The listing builds one solid part. Answer for the finished solid, in the listing's coordinates (mm). Face numbers are marked on the shaded views. A direction names the side the tool comes from. Round coordinates to 2 decimals unless told otherwise and drop trailing zeros. Order: outer loops, then holes, each group sorted by start corner. A loop starts at its lowest first (then second) coordinate and runs counter-clockwise, first axis right, second up. Notation, with made-up numbers: (-17.75, -38) - (38.25, -38) arc R13 ccw to (38.25, -26) - close; hole circle Ø10 at (-29.75, -34). An arc over 180 degrees is marked (long way). One line per item, written item: value. Start each with the question number.
1. A straight line is drawn through the part: line 1 (Z direction, x = 12, y = 18). Find the intervals that lie inside material, in ascending order.
2. Section A-A, the plane z = 11.5 is taken. Count the separate pieces of the cut face and the enclosed holes in it, then the cut area to 3 significant figures.
3. Section B-B, the plane x = 22 is taken. Give the vertices of the cut face in (y, z).
4. A tool of negligible diameter and unlimited length cuts with its end or side. For the marked faces 1, 2 and 3, from which of +Z, -Z, +X, -X, +Y, -Y can it reach the whole face along a straight path? Write none if from no direction.
5. Flat-ended cylindrical pins translate along their axes: P1, Ø3, axis at y = 20.5, z = 6.5, coming from the -X side; P2, Ø6, axis at y = 4, z = 10, coming from the +X side; P3, Ø0.6, axis at x = 3.5, z = 8, coming from the +Y side. Find the tip coordinate at first contact, or state that the pin passes through.
from build123d import *

# Parameters (mm, degrees)
F0_W     = 0.508
F0_H     = 27.8820712173
F1_DEPTH = 12.7
F0_W_2   = 29.972
F0_H_2   = 29.972
F2_DEPTH = 2.54


with BuildPart() as f1:
    # F0 (on Top) → F1 (new body)
    with BuildSketch(Plane.XY):
        with Locations((0.762, 15.0149643914)):
            Rectangle(F0_W, F0_H)
    extrude(amount=F1_DEPTH)



with BuildPart() as f1b:
    # F0 (on Top) → F1, piece 2 (new body)
    with BuildSketch(Plane.XY):
        with Locations((3.302, 15.0149643914)):
            Rectangle(F0_W, F0_H)
    extrude(amount=F1_DEPTH)


with BuildPart() as f1c:
    # F0 (on Top) → F1, piece 3 (new body)
    with BuildSketch(Plane.XY):
        with Locations((5.842, 15.0149643914)):
            Rectangle(F0_W, F0_H)
    extrude(amount=F1_DEPTH)


with BuildPart() as f1d:
    # F0 (on Top) → F1, piece 4 (new body)
    with BuildSketch(Plane.XY):
        with Locations((8.382, 15.0149643914)):
            Rectangle(F0_W, F0_H)
    extrude(amount=F1_DEPTH)


with BuildPart() as f1e:
    # F0 (on Top) → F1, piece 5 (new body)
    with BuildSketch(Plane.XY):
        with Locations((10.922, 15.0149643914)):
            Rectangle(F0_W, F0_H)
    extrude(amount=F1_DEPTH)


with BuildPart() as f1f:
    # F0 (on Top) → F1, piece 6 (new body)
    with BuildSketch(Plane.XY):
        with Locations((13.462, 15.0149643914)):
            Rectangle(F0_W, F0_H)
    extrude(amount=F1_DEPTH)


with BuildPart() as f1g:
    # F0 (on Top) → F1, piece 7 (new body)
    with BuildSketch(Plane.XY):
        with Locations((16.002, 15.0149643914)):
            Rectangle(F0_W, F0_H)
    extrude(amount=F1_DEPTH)


with BuildPart() as f1h:
    # F0 (on Top) → F1, piece 8 (new body)
    with BuildSketch(Plane.XY):
        with Locations((18.542, 15.0149643914)):
            Rectangle(F0_W, F0_H)
    extrude(amount=F1_DEPTH)


with BuildPart() as f1i:
    # F0 (on Top) → F1, piece 9 (new body)
    with BuildSketch(Plane.XY):
        with Locations((21.082, 15.0149643914)):
            Rectangle(F0_W, F0_H)
    extrude(amount=F1_DEPTH)


with BuildPart() as f1j:
    # F0 (on Top) → F1, piece 10 (new body)
    with BuildSketch(Plane.XY):
        with Locations((23.622, 15.0149643914)):
            Rectangle(F0_W, F0_H)
    extrude(amount=F1_DEPTH)


with BuildPart() as f1k:
    # F0 (on Top) → F1, piece 11 (new body)
    with BuildSketch(Plane.XY):
        with Locations((26.162, 15.0149643914)):
            Rectangle(F0_W, F0_H)
    extrude(amount=F1_DEPTH)


with BuildPart() as f1l:
    # F0 (on Top) → F1, piece 12 (new body)
    with BuildSketch(Plane.XY):
        with Locations((28.702, 15.0149643914)):
            Rectangle(F0_W, F0_H)
    extrude(amount=F1_DEPTH)


with BuildPart() as f1_1:
    add(f1.part)

    add(f1b.part)  # F2 merges F1b

    add(f1c.part)  # F2 merges F1c

    add(f1d.part)  # F2 merges F1d

    add(f1e.part)  # F2 merges F1e

    add(f1f.part)  # F2 merges F1f

    add(f1g.part)  # F2 merges F1g

    add(f1h.part)  # F2 merges F1h

    add(f1i.part)  # F2 merges F1i

    add(f1j.part)  # F2 merges F1j

    add(f1k.part)  # F2 merges F1k

    add(f1l.part)  # F2 merges F1l
    # F0 (on Top) → F2 (join)
    with BuildSketch(Plane.XY):
        with Locations((14.986, 14.986)):
            Rectangle(F0_W_2, F0_H_2)
        with Locations((0.762, 15.0149643914)):
            Rectangle(F0_W, F0_H, mode=Mode.SUBTRACT)
        with Locations((3.302, 15.0149643914)):
            Rectangle(F0_W, F0_H, mode=Mode.SUBTRACT)
        with Locations((5.842, 15.0149643914)):
            Rectangle(F0_W, F0_H, mode=Mode.SUBTRACT)
        with Locations((8.382, 15.0149643914)):
            Rectangle(F0_W, F0_H, mode=Mode.SUBTRACT)
        with Locations((10.922, 15.0149643914)):
            Rectangle(F0_W, F0_H, mode=Mode.SUBTRACT)
        with Locations((13.462, 15.0149643914)):
            Rectangle(F0_W, F0_H, mode=Mode.SUBTRACT)
        with Locations((16.002, 15.0149643914)):
            Rectangle(F0_W, F0_H, mode=Mode.SUBTRACT)
        with Locations((18.542, 15.0149643914)):
            Rectangle(F0_W, F0_H, mode=Mode.SUBTRACT)
        with Locations((21.082, 15.0149643914)):
            Rectangle(F0_W, F0_H, mode=Mode.SUBTRACT)
        with Locations((23.622, 15.0149643914)):
            Rectangle(F0_W, F0_H, mode=Mode.SUBTRACT)
        with Locations((26.162, 15.0149643914)):
            Rectangle(F0_W, F0_H, mode=Mode.SUBTRACT)
        with Locations((28.702, 15.0149643914)):
            Rectangle(F0_W, F0_H, mode=Mode.SUBTRACT)
    extrude(amount=F2_DEPTH)


solid = f1_1.part
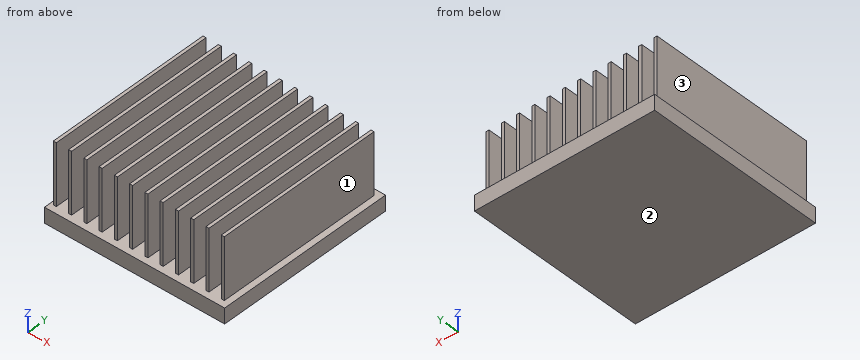
Answer list:
1. line 1: z = 0 to 2.54
2. separate pieces: 12
2. enclosed holes: 0
2. area: 170 mm²
3. outline: (0, 0) - (29.97, 0) - (29.97, 2.54) - (0, 2.54) - close
4. face 1: +Z, +X, +Y, -Y
4. face 2: -Z, +X, -X, +Y, -Y
4. face 3: +Z, -X, +Y, -Y
5. P1: stops at x = 0.51
5. P2: stops at x = 28.96
5. P3: stops at y = 28.96
